```python
from build123d import *

# Parameters (mm, degrees)
SKETCH1_W           = 53
SKETCH1_H           = 35
BOSS_EXTRUDE1_DEPTH = 15
SKETCH3_R           = 13
CUT_EXTRUDE1_DEPTH  = 50
BOSS_EXTRUDE4_START = -3
SKETCH6_R           = 13
BOSS_EXTRUDE4_DEPTH = 3
SKETCH7_R           = 4.5
CUT_EXTRUDE2_DEPTH  = 54
SKETCH10_R          = 2
CUT_EXTRUDE3_DEPTH  = 16
SKETCH17_R          = 1.75
CUT_EXTRUDE5_DEPTH  = 4


with BuildPart() as part:
    # Sketch1 → Boss-Extrude1 (new body)
    with BuildSketch(Plane.XY):
        Rectangle(SKETCH1_W, SKETCH1_H)
    extrude(amount=BOSS_EXTRUDE1_DEPTH)

    # Sketch3 → Cut-Extrude1 (cut)
    with BuildSketch(Plane(origin=(26.5, 0, 0), x_dir=(0, 0, -1), z_dir=(1, 0, 0))):
        Circle(SKETCH3_R)
    extrude(amount=-CUT_EXTRUDE1_DEPTH, mode=Mode.SUBTRACT)

    # Sketch6 → Boss-Extrude4 (add)
    with BuildSketch(Plane.ZY.offset(26.5).offset(BOSS_EXTRUDE4_START)):
        Circle(SKETCH6_R)
    extrude(amount=BOSS_EXTRUDE4_DEPTH)

    # Sketch7 → Cut-Extrude2 (cut, through all)
    with BuildSketch(Plane.ZY.offset(26.5)):
        Circle(SKETCH7_R)
    extrude(amount=-CUT_EXTRUDE2_DEPTH, mode=Mode.SUBTRACT)

    # Sketch10 → Cut-Extrude3 (cut, through all)
    with BuildSketch(Plane(origin=(0, 0, 0), x_dir=(-1, 0, 0), z_dir=(0, 0, -1))):
        with Locations((-17.5, 15.25)):
            Circle(SKETCH10_R)
        with Locations((17.5, 15.25)):
            Circle(SKETCH10_R)
        with Locations((17.5, -15.25)):
            Circle(SKETCH10_R)
        with Locations((-17.5, -15.25)):
            Circle(SKETCH10_R)
    extrude(amount=-CUT_EXTRUDE3_DEPTH, mode=Mode.SUBTRACT)

    # Sketch17 → Cut-Extrude5 (cut, through all)
    with BuildSketch(Plane(origin=(-23.5, 0, 0), x_dir=(0, 0, -1), z_dir=(1, 0, 0))):
        with Locations((0, -8.5)):
            Circle(SKETCH17_R)
        with Locations((0, 8.5)):
            Circle(SKETCH17_R)
    extrude(amount=-CUT_EXTRUDE5_DEPTH, mode=Mode.SUBTRACT)


solid = part.part
```
The model under review builds one solid part; all positions refer to its coordinate system, in mm. A direction names the side the tool comes from. Coordinates: 2 decimals unless noted, no trailing zeros. Write each loop counter-clockwise with the first axis right and the second up, starting at its lowest first coordinate (ties: lowest second). Pieces come first, ordered by that corner, then holes. Notation, with made-up numbers: (28, 57) -> (77, 57) arc R17 ccw to (77, 75) -> close; hole circle Ø5 at (53.5, 24.5). An arc over 180 degrees is marked (long way). One line per item, written item: value. Start each with the question number.
Q1. To check wall thickness, follow probe 1 along Y at (x, z) = (-17.5, 0.5); probe 2 along Y at (x, z) = (18, 14); probe 3 along Y at (x, z) = (16, 3). State the ranges of each line that lie inside material, in increasing order.
Q2. Add section A-A, the plane x = -17.5. Give the boundary of the cut face in (y, z).
Q3. Clearance check with flat-ended pins moving along their axes: P1, Ø2.5, axis at x = -17.5, y = 15.25, coming from the -Z side; P2, Ø3.5, axis at x = 4, y = 16, coming from the -Z side; P3, Ø10.5, axis at y = 0, z = 0, coming from the -X side. State where each tip first meets the part, or that it passes through.
Q4. Add section D-D, the plane z = 6.25. Give the boundary of the cut face in (x, y).
Q5. Add section C-C, the plane y = -3. Give the boundary of the cut face in (x, z).
Q6. The part is to be moulded in two halves that separate along X. For faces 4 (the face through (-25, -7, -0.9)), 5 (the face through (17.76, 17.233, 7.395)), 6 (the face through (-23.5, 0, 6)), 7 (the face through (-26.5, 0, 7)), say which applies: +X half, -X half, draft (parallel to the pull), parting line (faces both ways), or undercut.
Q7. Add section B-B, the plane y = 15.25. Give the boundary of the cut face in (x, z).
Q8. For faces 1 (the face through (0, 15, 0)), 2 (the face through (0, -15, 0)), 3 (the face through (2, 0, 13)), list the 3-axis set-ups (+Z, -Z, +X, -X, +Y, -Y) from which the entire face can be reached by the end or side of a thin tool; tool diameter is ignored.
Response:
1. probe 1: -17.5 to -17.25, -13.25 to -12.99, 12.99 to 13.25, 17.25 to 17.5
1. probe 2: -17.5 to -17.19, -13.31 to 13.31, 17.19 to 17.5
1. probe 3: -17.5 to -16.57, -13.93 to -12.65, 12.65 to 13.93, 16.57 to 17.5
2. outline: (-17.5, 0) -> (-17.25, 0) -> (-17.25, 15) -> (-17.5, 15) -> close; (-13.25, 0) -> (-13, 0) arc R13 cw to (13, 0) -> (13.25, 0) -> (13.25, 15) -> (-13.25, 15) -> close; (17.25, 0) -> (17.5, 0) -> (17.5, 15) -> (17.25, 15) -> close
3. P1: through
3. P2: z = 0
3. P3: x = -26.5
4. outline: (-26.5, -17.5) -> (26.5, -17.5) -> (26.5, -11.4) -> (-23.5, -11.4) -> (-23.5, 11.4) -> (26.5, 11.4) -> (26.5, 17.5) -> (-26.5, 17.5) -> close; hole circle Ø4 at (-17.5, -15.25); hole circle Ø4 at (-17.5, 15.25); hole circle Ø4 at (17.5, -15.25); hole circle Ø4 at (17.5, 15.25)
5. outline: (-26.5, -12.65) -> (-23.5, -12.65) -> (-23.5, -3.35) -> (-26.5, -3.35) -> close; (-26.5, 3.35) -> (-23.5, 3.35) -> (-23.5, 12.65) -> (26.5, 12.65) -> (26.5, 15) -> (-26.5, 15) -> close
6. face 4: draft
6. face 5: undercut
6. face 6: +X half
6. face 7: -X half
7. outline: (-26.5, 0) -> (-19.5, 0) -> (-19.5, 15) -> (-26.5, 15) -> close; (-15.5, 0) -> (15.5, 0) -> (15.5, 15) -> (-15.5, 15) -> close; (19.5, 0) -> (26.5, 0) -> (26.5, 15) -> (19.5, 15) -> close
8. face 1: -Z, +X, -X, +Y
8. face 2: -Z, +X, -X, -Y
8. face 3: -Z, +X
